from build123d import *

# Parameters (mm, degrees)
SKETCH1_R           = 18
BOSS_EXTRUDE1_DEPTH = 13.3
SKETCH2_R           = 11
BOSS_EXTRUDE2_DEPTH = 2
SKETCH4_R           = 1.5
CUT_EXTRUDE1_DEPTH  = 39.287857083
SKETCH5_R           = 4
BOSS_EXTRUDE3_DEPTH = 16
CUT_EXTRUDE2_DEPTH  = 15


with BuildPart() as part:
    # Sketch1 → Boss-Extrude1 (new, symmetric)
    with BuildSketch(Plane(origin=(0, 0, 0), x_dir=(1, 0, 0), z_dir=(0, 1, 0))):
        with Locations(Location((0, 0, 0), (0, 0, 270))):
            Circle(SKETCH1_R)
    extrude(amount=BOSS_EXTRUDE1_DEPTH, both=True)

    # Sketch2 → Boss-Extrude2 (add)
    with BuildSketch(Plane(origin=(0, 13.3, 0), x_dir=(1, 0, 0), z_dir=(0, 1, 0))):
        with Locations(Location((0, 0, 0), (0, 0, 270))):
            Circle(SKETCH2_R)
    extrude(amount=BOSS_EXTRUDE2_DEPTH)

    # Sketch4 → Cut-Extrude1 (cut, through all)
    with BuildSketch(Plane(origin=(0, 15.3, 0), x_dir=(1, 0, 0), z_dir=(0, 1, 0))):
        with Locations(Location((-14, 0, 0), (0, 0, 270))):
            Circle(SKETCH4_R)
        with Locations(Location((0, -14, 0), (0, 0, 270))):
            Circle(SKETCH4_R)
        with Locations(Location((14, 0, 0), (0, 0, 270))):
            Circle(SKETCH4_R)
        with Locations(Location((0, 14, 0), (0, 0, 270))):
            Circle(SKETCH4_R)
    extrude(amount=-CUT_EXTRUDE1_DEPTH, mode=Mode.SUBTRACT)

    # Sketch5 → Boss-Extrude3 (add)
    with BuildSketch(Plane(origin=(0, 15.3, 0), x_dir=(1, 0, 0), z_dir=(0, 1, 0))):
        with Locations(Location((0, 0, 0), (0, 0, 270))):
            Circle(SKETCH5_R)
    extrude(amount=BOSS_EXTRUDE3_DEPTH)

    # Sketch6 → Cut-Extrude2 (cut)
    with BuildSketch(Plane(origin=(0, 31.3, 0), x_dir=(1, 0, 0), z_dir=(0, 1, 0))):
        with BuildLine():
            Line((-3, -4), (-3, 4))
            ThreePointArc((-3, 4), (-5, 0), (-3, -4))
        make_face()
        with BuildLine():
            Line((3, -4), (3, 4))
            ThreePointArc((3, 4), (5, 0), (3, -4))
        make_face()
    extrude(amount=-CUT_EXTRUDE2_DEPTH, mode=Mode.SUBTRACT)


solid = part.part
Input: part model. Units: mm. Frame: model coordinates. A direction names the side the tool comes from. Round coordinates to 2 decimals unless told otherwise and drop trailing zeros. Loops run counter-clockwise (first coordinate to the right, second up) from the corner with the lowest first, then second, coordinate; pieces in that order, holes last. Notation, with made-up numbers: M -0.5,-21 L 7.5,-21 A14 cw 7.5,-16 Z; hole C -26,-15.5 d8. An arc over 180 degrees is marked long. Answer as CSV lines item,"result". Start each with the question number.
(1) Section D-D, the plane z = 14. Output: boundary loops of the cut face in (x, y), plus the area to 3 significant figures.
(2) Section A-A, the plane z = 0. Output: boundary loops of the cut face in (x, y), plus the area to 3 significant figures.
(3) Reachability of faces 1 (the flat face through (3, 24, 0)), 2 (the cylindrical face through (14.45, 0.19, 1.43)), 3 (the flat face through (0, 31.3, 0)), 4 (the flat face through (-3, 24, 0)), 5 (the cylindrical face through (0, 23, -4)) from +Z, -Z, +X, -X, +Y, -Y: full face, straight path, thin tool, end or side. Return the list, or none.
(4) First-contact query: pin 1 (2.5 mm diameter, centred on y = 25, z = 1, fed in from -X); pin 2 (2.5 mm diameter, centred on y = 26, z = -0.5, fed in from +X); pin 3 (4 mm diameter, centred on x = 0, z = -14, fed in from +Y); pin 4 (1.1 mm diameter, centred on x = -3.5, z = -0.5, fed in from +Y). Flat tips, straight axial feed; report the tip coordinate or a pass-through.
(5) Section B-B, the plane x = -14. Output: boundary loops of the cut face in (y, z).
(6) Draft query along X for faces 6 (the cylindrical face through (5.407, 0.186, 17.169)), 7 (the cylindrical face through (0.07, 0.19, -15.5)), 8 (the flat face through (-8, 13.3, -8)). Return one class per face: released by +X, released by -X, zero draft, split by the parting line, or undercut.
(7) Line query: line 1 (X direction, y = 3, z = 0); line 2 (Y direction, x = -9.5, z = 2); line 3 (Y direction, x = 7, z = 14). Output: solid intervals per line, ascending. Write a range as [from, to].
(8) Section C-C, the plane y = 6.5. Output: boundary loops of the cut face in (x, z), plus the area to 3 significant figures.
Values found:
1,outline,"M -11.31,-13.3 L -1.5,-13.3 L -1.5,13.3 L -11.31,13.3 Z; M 1.5,-13.3 L 11.31,-13.3 L 11.31,13.3 L 1.5,13.3 Z"
1,area,"522 mm²"
2,outline,"M -18,-13.3 L -15.5,-13.3 L -15.5,13.3 L -18,13.3 Z; M -12.5,-13.3 L 12.5,-13.3 L 12.5,13.3 L 11,13.3 L 11,15.3 L 4,15.3 L 4,16.3 L 3,16.3 L 3,31.3 L -3,31.3 L -3,16.3 L -4,16.3 L -4,15.3 L -11,15.3 L -11,13.3 L -12.5,13.3 Z; M 15.5,-13.3 L 18,-13.3 L 18,13.3 L 15.5,13.3 Z"
2,area,"940 mm²"
3,face 1,"+Z, -Z, +X, +Y"
3,face 2,"+Y, -Y"
3,face 3,"+Z, -Z, +X, -X, +Y"
3,face 4,"+Z, -Z, -X, +Y"
3,face 5,"+Y"
4,pin 1,"stops at x = -3"
4,pin 2,"stops at x = 3"
4,pin 3,"stops at y = 13.3"
4,pin 4,"stops at y = 31.3"
5,outline,"M -13.3,-11.31 L 13.3,-11.31 L 13.3,-1.5 L -13.3,-1.5 Z; M -13.3,1.5 L 13.3,1.5 L 13.3,11.31 L -13.3,11.31 Z"
6,face 6,"split by the parting line"
6,face 7,"undercut"
6,face 8,"zero draft"
7,line 1,"x = [-18, -15.5], [-12.5, 12.5], [15.5, 18]"
7,line 2,"y = [-13.3, 15.3]"
7,line 3,"y = [-13.3, 13.3]"
8,outline,"C 0,0 d36; hole C -14,0 d3; hole C 0,-14 d3; hole C 0,14 d3; hole C 14,0 d3"
8,area,"990 mm²"
